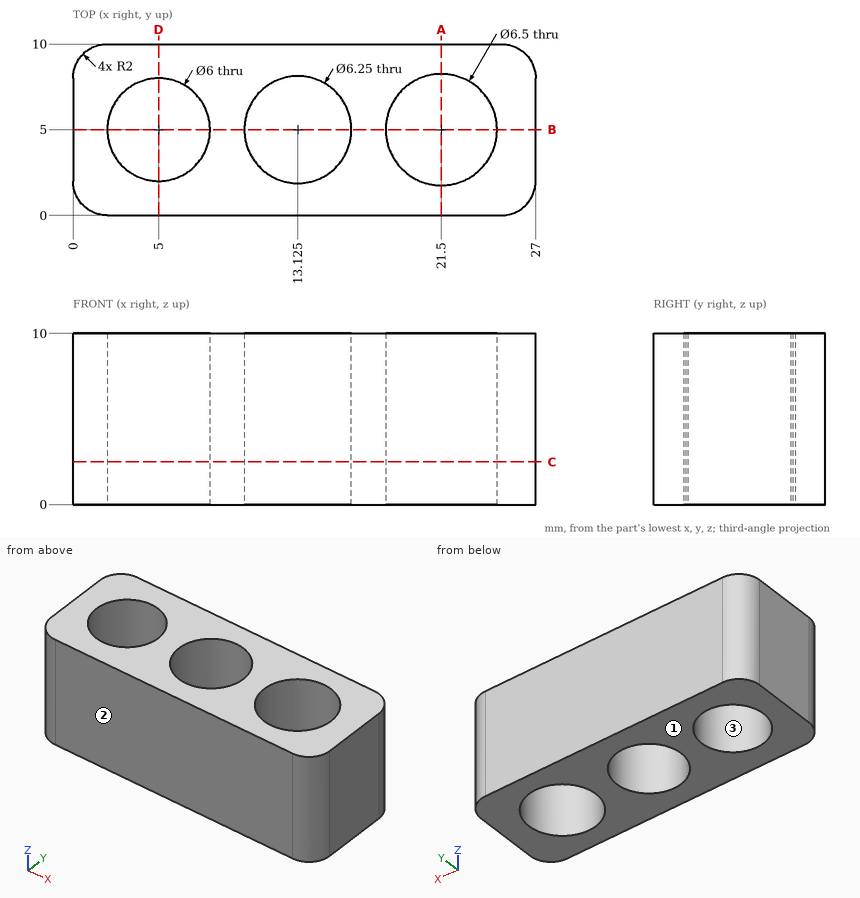
Study the drawing (mm; zero at the part's minimum x, y, z) and answer. Coordinates: 2 decimals unless noted, no trailing zeros. Loops run counter-clockwise (first coordinate to the right, second up) from the corner with the lowest first, then second, coordinate; pieces in that order, holes last. Notation, with made-up numbers: M -18,70 L 20,70 A15 ccw 20,85 Z; hole C 0,49 d7. An arc over 180 degrees is marked long. Answer in a Markdown table with one row per item. Add a question column.
1. Consider L1, parallel to Y at x = 21.5, z = 3.5; L2, parallel to X at y = 6, z = 8.25; L3, parallel to Y at x = 14, z = 9. Determine where each line is inside the solid, lowest interval first.
2. Flat-ended cylindrical pins translate along their axes: P1, Ø5, axis at y = 8, z = 7.5, coming from the -X side; P2, Ø5, axis at x = 5, y = 5, coming from the -Z side. Find the tip coordinate at first contact, or state that the pin passes through.
3. Find section D-D, the plane x = 5. Write down the section's boundary in (y, z).
4. Find section C-C, the plane z = 2.5. Write down the section's boundary in (x, y) (3 decimals), then the cut area to 3 significant figures.
5. Find section A-A, the plane x = 21.5. Write down the section's boundary in (y, z), then the cut area to 3 significant figures.
6. Find section B-B, the plane y = 5. Write down the section's boundary in (x, z).
7. The mould has two halves that part along Y. Classify the marked faces 1, 2 and 3: pulls with the +Y half, pulls with the -Y half, needs draft (parallel to the pull), parting line crosses it, or undercut.
Reported:
| question | item | result |
|---|---|---|
| 1 | L1 | y = 0 to 1.75, 8.25 to 10 |
| 1 | L2 | x = 0 to 2.17, 7.83 to 10.16, 16.09 to 18.41, 24.59 to 27 |
| 1 | L3 | y = 0 to 2, 8 to 10 |
| 2 | P1 | stops at x = 0 |
| 2 | P2 | passes through |
| 3 | outline | M 0,0 L 2,0 L 2,10 L 0,10 Z; M 8,0 L 10,0 L 10,10 L 8,10 Z |
| 4 | outline | M 0,2 A2 ccw 2,0 L 25,0 A2 ccw 27,2 L 27,8 A2 ccw 25,10 L 2,10 A2 ccw 0,8 Z; hole C 5,5 d6; hole C 13.125,5 d6.25; hole C 21.5,5 d6.5 |
| 4 | area | 174 mm^2 |
| 5 | outline | M 0,0 L 1.75,0 L 1.75,10 L 0,10 Z; M 8.25,0 L 10,0 L 10,10 L 8.25,10 Z |
| 5 | area | 35.0 mm^2 |
| 6 | outline | M 0,0 L 2,0 L 2,10 L 0,10 Z; M 8,0 L 10,0 L 10,10 L 8,10 Z; M 16.25,0 L 18.25,0 L 18.25,10 L 16.25,10 Z; M 24.75,0 L 27,0 L 27,10 L 24.75,10 Z |
| 7 | face 1 | needs draft |
| 7 | face 2 | pulls with the -Y half |
| 7 | face 3 | undercut |
